Source: CAD feature listing. Evaluate the final solid. Frame: model axes, mm. Face numbers are marked on the shaded views. A direction names the side the tool comes from. Give positions to 0.01 mm unless a question says otherwise; leave off trailing zeros. Write each loop counter-clockwise with the first axis right and the second up, starting at its lowest first coordinate (ties: lowest second). Pieces come first, ordered by that corner, then holes. Notation, with made-up numbers: (-21.5, 34.25) - (15.5, 34.25) arc R8 ccw to (15.5, 49.25) - close; hole circle Ø7 at (-7, -3). An arc over 180 degrees is marked (long way). One line per question, with ' | ' between items. Start each with the question number.
(1) Pin query (flat end, axial travel): pin 1 (0.6 mm diameter, centred on y = 7, z = 5.5, fed in from +X); pin 2 (1 mm diameter, centred on y = 6.5, z = 4.5, fed in from -X); pin 3 (2 mm diameter, centred on y = 15, z = 5.5, fed in from -X); pin 4 (2 mm diameter, centred on x = 25.5, y = 9.5, fed in from +Z). Return the tip coordinate at first contact, or that it passes through.
(2) Section C-C, the plane x = 35.56. Return loops of the section in (y, z) (3 decimals), plus the area to 3 significant figures.
(3) Section D-D, the plane x = 14. Return loops of the section in (y, z).
(4) Access query for the marked faces 1, 2, 3, 4 and 5. Directions: +Z, -Z, +X, -X, +Y, -Y. A direction counts if a zero-diameter tool reaches every point of the face in a straight line with its end or side. Return the directions, or none.
(5) Ray query, line 1 (Y direction, x = 35.56, z = 0.3) (3 decimals); line 2 (Y direction, x = 23, z = 4.75); line 3 (Y direction, x = 20, z = 3). Return the intervals inside material, ascending. Write a range as [from, to].
(6) Section B-B, the plane y = 2.54. Return loops of the section in (x, z) (3 decimals), plus the area to 3 significant figures.
(7) Draft query along X for the marked faces 6, 7 and 8. Return one class per face: +X half, -X half, draft (parallel to the pull), parting line (faces both ways), or undercut.
(8) Section A-A, the plane z = 1.5. Return loops of the section in (x, y), plus the area to 3 significant figures.
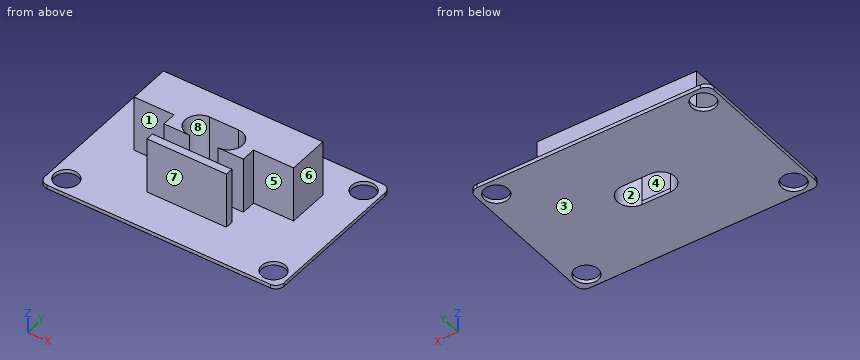
```python
from build123d import *

# Parameters (mm, degrees)
SKETCH1_W           = 38.1
SKETCH1_H           = 25.4
BOSS_EXTRUDE1_DEPTH = 0.6
SKETCH2_W           = 25.4
SKETCH2_H           = 12.7
BOSS_EXTRUDE2_DEPTH = 8.89
CUT_EXTRUDE1_DEPTH  = 25.4
CUT_EXTRUDE2_DEPTH  = 8.89
SKETCH5_R           = 1.905
CUT_EXTRUDE4_DEPTH  = 5.08
FILLET4_R           = 1.27


with BuildPart() as part:
    # Sketch1 → Boss-Extrude1 (new body)
    with BuildSketch(Plane.XY):
        with Locations((19.05, 12.7)):
            Rectangle(SKETCH1_W, SKETCH1_H)
    extrude(amount=BOSS_EXTRUDE1_DEPTH)

    # Sketch2 → Boss-Extrude2 (add)
    with BuildSketch(Plane.XY.offset(0.6)):
        with Locations((19.05, 12.7)):
            Rectangle(SKETCH2_W, SKETCH2_H)
    extrude(amount=BOSS_EXTRUDE2_DEPTH)

    # Sketch3 → Cut-Extrude1 (cut)
    with BuildSketch(Plane.XY.offset(9.49)):
        with BuildLine():
            Line((21.336, 14.732), (16.764, 14.732))
            ThreePointArc((16.764, 14.732), (14.478, 12.446), (16.764, 10.16))
            Line((16.764, 10.16), (21.336, 10.16))
            ThreePointArc((21.336, 10.16), (23.622, 12.446), (21.336, 14.732))
        make_face()
    extrude(amount=-CUT_EXTRUDE1_DEPTH, mode=Mode.SUBTRACT)

    # Sketch3<3> → Cut-Extrude2 (cut)
    with BuildSketch(Plane.XY.offset(9.49)):
        Polygon((21.336, 10.16), (16.764, 10.16), (12.707051154, 10.16), (12.707051154, 12.446), (6.35, 12.446), (6.35, 6.35), (12.707051154, 6.35), (12.707051154, 7.579234478), (25.362079922, 7.579234478), (25.362079922, 6.35), (31.75, 6.35), (31.75, 12.446), (25.362079922, 12.446), (25.362079922, 10.16), align=None)
    extrude(amount=-CUT_EXTRUDE2_DEPTH, mode=Mode.SUBTRACT)

    # Sketch5 → Cut-Extrude4 (cut)
    with BuildSketch(Plane.XY.offset(0.6)):
        with Locations((2.54, 22.86)):
            Circle(SKETCH5_R)
        with Locations(Location((35.56, 22.86, 0), (0, 0, 180))):
            Circle(SKETCH5_R)
        with Locations(Location((2.54, 2.54, 0), (0, 0, 180))):
            Circle(SKETCH5_R)
        with Locations((35.56, 2.54)):
            Circle(SKETCH5_R)
    extrude(amount=-CUT_EXTRUDE4_DEPTH, mode=Mode.SUBTRACT)

    # Fillet4
    fillet4_edges = [part.edges().sort_by_distance(p)[0] for p in [
        (0, 0, 0.3),
        (38.1, 0, 0.3),
        (38.1, 25.4, 0.3),
        (0, 25.4, 0.3),
    ]]
    fillet(fillet4_edges, radius=FILLET4_R)


solid = part.part
```
Check sheet entries:
1) pin 1: x = 25.36 | pin 2: x = 12.71 | pin 3: x = 6.35 | pin 4: z = 9.49
2) outline: (0, 0) - (0.635, 0) - (0.635, 0.6) - (0, 0.6) - close; (4.445, 0) - (20.955, 0) - (20.955, 0.6) - (4.445, 0.6) - close; (24.765, 0) - (25.4, 0) - (25.4, 0.6) - (24.765, 0.6) - close | area: 10.7 mm²
3) outline: (0, 0) - (25.4, 0) - (25.4, 0.6) - (19.05, 0.6) - (19.05, 9.49) - (10.16, 9.49) - (10.16, 0.6) - (7.58, 0.6) - (7.58, 9.49) - (6.35, 9.49) - (6.35, 0.6) - (0, 0.6) - close
4) face 1: +Z, -X, -Y | face 2: +Z, -Z | face 3: -Z, +X, -X, +Y, -Y | face 4: +Z, +X, -X | face 5: +Z, +X, -Y
5) line 1: [0, 0.635], [4.445, 20.955], [24.765, 25.4] | line 2: [6.35, 7.58], [10.16, 10.88], [14.01, 19.05] | line 3: [6.35, 7.58], [14.73, 19.05]
6) outline: (0, 0) - (0.635, 0) - (0.635, 0.6) - (0, 0.6) - close; (4.445, 0) - (33.655, 0) - (33.655, 0.6) - (4.445, 0.6) - close; (37.465, 0) - (38.1, 0) - (38.1, 0.6) - (37.465, 0.6) - close | area: 18.3 mm²
7) face 6: +X half | face 7: draft | face 8: undercut
8) outline: (6.35, 12.45) - (12.71, 12.45) - (12.71, 10.16) - (16.76, 10.16) arc R2.29 cw to (16.76, 14.73) - (21.34, 14.73) arc R2.29 cw to (21.34, 10.16) - (25.36, 10.16) - (25.36, 12.45) - (31.75, 12.45) - (31.75, 19.05) - (6.35, 19.05) - close; (12.71, 6.35) - (25.36, 6.35) - (25.36, 7.58) - (12.71, 7.58) - close | area: 175 mm²
